Can you work these out from the drawing? Everything is in mm from the part's minimum corner. A direction names the side the tool comes from. Give positions to 0.01 mm unless a question says otherwise; leave off trailing zeros. Order: outer loops, then holes, each group sorted by start corner. A loop starts at its lowest first (then second) coordinate and runs counter-clockwise, first axis right, second up. Notation, with made-up numbers: M -22.75,39.5 L 14.25,39.5 A21 cw 14.25,78.5 Z; hole C 79,56.5 d11. An arc over 180 degrees is marked long. Use a Markdown table: item, result. Add a question column.
Item 1: Suppose I cut it at B-B on y = 12.5. Write out the boundary of the cut face in (x, z).
Item 2: Suppose I cut it at A-A on x = 8.5. Write out the boundary of the cut face in (y, z), plus the area to 3 significant figures.
Item 3: For the marked faces 1, 2 and 3, which set-ups out of +Z, -Z, +X, -X, +Y, -Y let a thin tool reach every point of the face, with its end or its side?
Item 4: Suppose I cut it at D-D on x = 14.25. Write out the boundary of the cut face in (y, z).
Item 5: If I drill on L1, parallel to Z at x = 7.5, y = 1; L2, parallel to Z at x = 3, y = 11; L3, parallel to Y at x = 8, z = 16.5, over which ranges is the centre line in solid material (lowest first)? Write a range as from..to.
Item 6: Suppose I cut it at C-C on z = 19.25. Write out the boundary of the cut face in (x, y), plus the area to 3 significant figures.
Item 7: I'm going to push flat-ended pins straight in: pin 1 Ø8 at (y, z) = (4.5, 11) entering from -X; pin 2 Ø10 at (x, y) = (15, 7.5) entering from +Z; pin 3 Ø4 at (x, z) = (4, 17) entering from +Y; pin 4 Ø8 at (x, y) = (5.5, 17) entering from +Z. Where does each tip first touch, or does it pass through?
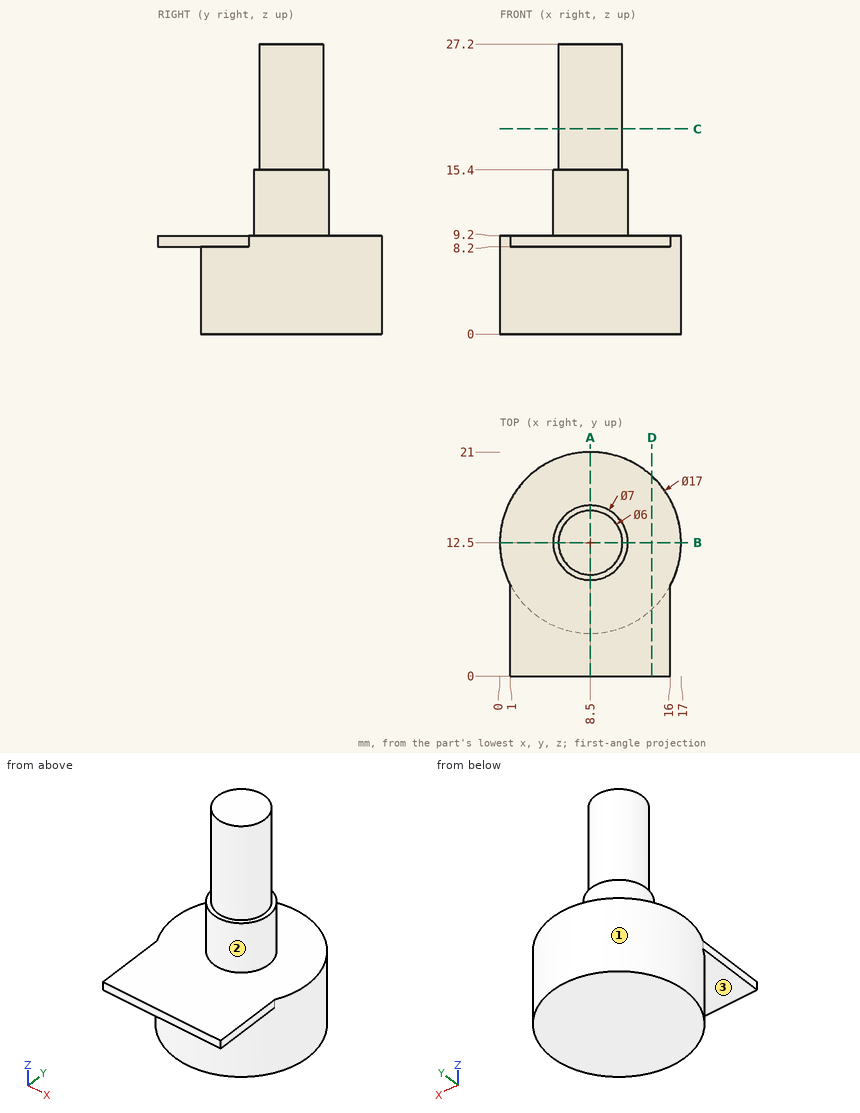
Findings below:
| question | item | result |
|---|---|---|
| 1 | outline | M 0,0 L 17,0 L 17,9.2 L 12,9.2 L 12,15.4 L 11.5,15.4 L 11.5,27.2 L 5.5,27.2 L 5.5,15.4 L 5,15.4 L 5,9.2 L 0,9.2 Z |
| 2 | outline | M 0,8.2 L 4,8.2 L 4,0 L 21,0 L 21,9.2 L 16,9.2 L 16,15.4 L 15.5,15.4 L 15.5,27.2 L 9.5,27.2 L 9.5,15.4 L 9,15.4 L 9,9.2 L 0,9.2 Z |
| 2 | area | 275 mm^2 |
| 3 | face 1 | -Z |
| 3 | face 2 | +Z |
| 3 | face 3 | -Z, -Y |
| 4 | outline | M 0,8.2 L 6.24,8.2 L 6.24,0 L 18.76,0 L 18.76,9.2 L 0,9.2 Z |
| 5 | L1 | z = 8.2..9.2 |
| 5 | L2 | z = 0..9.2 |
| 5 | L3 | y = 9.54..15.46 |
| 6 | outline | C 8.5,12.5 d6 |
| 6 | area | 28.3 mm^2 |
| 7 | pin 1 | stops at x = 1 |
| 7 | pin 2 | stops at z = 15.4 |
| 7 | pin 3 | stops at y = 14.16 |
| 7 | pin 4 | stops at z = 27.2 |
